```python
from build123d import *

# Parameters (mm, degrees)
SKETCH001_R     = 2.15
POCKET_DEPTH    = 3.119566
CHAMFER_SIZE    = 0.25
CHAMFER001_SIZE = 0.2


with BuildPart() as pocket:
    # Sketch003 → Revolution001 (revolve)
    with BuildSketch(Plane.XZ):
        Polygon((0, -2.118566), (1.15, -1.7), (1.15, 1), (0, 1), align=None)
    revolve(axis=Axis((0, 0, 0), (0, 0, 1)))

    # Sketch001 (on Face3 of Revolution001) → Pocket (cut, through all)
    with BuildSketch(Plane(origin=(0, 0, 1), x_dir=(-1, 0, 0), z_dir=(0, 0, 1))):
        Circle(SKETCH001_R)
        Polygon((-0.57735, 1), (0.57735, 1), (1.154701, 0), (0.57735, -1), (-0.57735, -1), (-1.154701, 0), align=None, mode=Mode.SUBTRACT)
    extrude(amount=-POCKET_DEPTH, mode=Mode.SUBTRACT)


with BuildPart() as chamfer001:
    # Sketch → Revolution (revolve)
    with BuildSketch(Plane.XZ):
        Polygon((1.15, 0), (3.199999, 0), (1.5, -1.7), (1.5, -30), (0, -30), (0, -1.150001), align=None)
    revolve(axis=Axis((0, 0, 0), (0, 0, 1)))

    # Cut: cut Pocket
    add(pocket.part, mode=Mode.SUBTRACT)

    # Chamfer
    chamfer_edges = [chamfer001.edges().sort_by_distance(p)[0] for p in [
        (-3.199999, 0, 0),
    ]]
    chamfer(chamfer_edges, length=CHAMFER_SIZE)

    # Chamfer001
    chamfer001_edges = [chamfer001.edges().sort_by_distance(p)[0] for p in [
        (-1.5, 0, -30),
    ]]
    chamfer(chamfer001_edges, length=CHAMFER001_SIZE)


solid = chamfer001.part
```
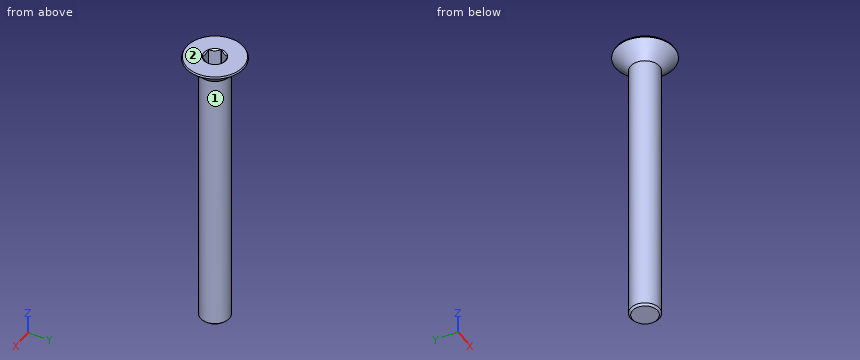
Work out the finished part from the listing and answer in its coordinate system (mm). Face numbers are marked on the shaded views. A direction names the side the tool comes from. Give positions to 0.01 mm unless a question says otherwise; leave off trailing zeros. Order: outer loops, then holes, each group sorted by start corner. A loop starts at its lowest first (then second) coordinate and runs counter-clockwise, first axis right, second up.
1. Each of these flat-tipped pins is pushed along its axis until it touches: P1, Ø2, axis at x = -1.5, z = -20, coming from the +Y side; P2, Ø1.5, axis at x = -2, z = -16, coming from the +Y side; P3, Ø1.2, axis at x = 0, z = -1.5, coming from the -Y side. Where does it stop, or does it pass through?
Result sheet:
P1: stops at y = 1.41
P2: stops at y = 0.83
P3: stops at y = -2.3
2. Section A-A, the plane z = -2.75 is taken. Determine the outline of the cut face in (x, y), and give its area (3 significant figures).
Result sheet:
outline: circle Ø3 at (0, 0)
area: 7.07 mm2
3. Straight lines are drawn through the part: L1, parallel to Z at x = 0.75, y = -2.5; L2, parallel to Y at x = 0, z = -13.75; L3, parallel to X at y = -0.5, z = -18. For each, find the intervals that lie inside material, in ascending order.
Result sheet:
L1: z = -0.59 to 0
L2: y = -1.5 to 1.5
L3: x = -1.41 to 1.41
4. For the marked faces 1 and 2, determine the directions among +Z, -Z, +X, -X, +Y, -Y from which every point of the face is accessible in a straight line to the end or side of a thin tool.
Result sheet:
face 1: -Z
face 2: +Z, +X, -X, +Y, -Y
